from build123d import *

# Parameters (mm, degrees)
SKETCH1_R                      = 6.25
SKETCH1_R_2                    = 3.75
SKETCH1_R_3                    = 2.5
BOSS_EXTRUDE1_DEPTH            = 5
SKETCH2_R                      = 4
BOSS_EXTRUDE2_DEPTH            = 22.5
SKETCH3_R                      = 3
BOSS_EXTRUDE3_DEPTH            = 2
SKETCH4_R                      = 4
BOSS_EXTRUDE4_DEPTH            = 2
SKETCH6_W                      = 1.89865
SKETCH6_H                      = 5
F_6_CLEARANCE_HOLE1_AT_2_COUNT = 2
F_6_CLEARANCE_HOLE1_AT_2_PITCH = 7.75


with BuildPart() as part:
    # Sketch1 → Boss-Extrude1 (new body)
    # profile 1 of 15: a face of its own
    with BuildSketch(Plane(origin=(0, 0, 0), x_dir=(1, 0, 0), z_dir=(0, 1, 0))):
        Circle(SKETCH1_R)
    # profile 2 of 15: a face of its own
    with BuildSketch(Plane(origin=(0, 0, 0), x_dir=(1, 0, 0), z_dir=(0, 1, 0))):
        with Locations((-7.75, 0)):
            Circle(SKETCH1_R_2)
        with Locations((-7.75, 0)):
            Circle(SKETCH1_R_3, mode=Mode.SUBTRACT)
    # profile 3 of 15: a face of its own
    with BuildSketch(Plane(origin=(0, 0, 0), x_dir=(1, 0, 0), z_dir=(0, 1, 0))):
        Circle(SKETCH1_R)
    # profile 4 of 15: a face of its own
    with BuildSketch(Plane(origin=(0, 0, 0), x_dir=(1, 0, 0), z_dir=(0, 1, 0))):
        with Locations((-7.75, 0)):
            Circle(SKETCH1_R_2)
        with Locations((-7.75, 0)):
            Circle(SKETCH1_R_3, mode=Mode.SUBTRACT)
    # profile 5 of 15: a face of its own
    with BuildSketch(Plane(origin=(0, 0, 0), x_dir=(1, 0, 0), z_dir=(0, 1, 0))):
        with Locations((7.75, 0)):
            Circle(SKETCH1_R_2)
    # profile 6 of 15: a face of its own
    with BuildSketch(Plane(origin=(0, 0, 0), x_dir=(1, 0, 0), z_dir=(0, 1, 0))):
        Circle(SKETCH1_R)
    # profile 7 of 15: a face of its own
    with BuildSketch(Plane(origin=(0, 0, 0), x_dir=(1, 0, 0), z_dir=(0, 1, 0))):
        with Locations((-7.75, 0)):
            Circle(SKETCH1_R_2)
    # profile 8 of 15: a face of its own
    with BuildSketch(Plane(origin=(0, 0, 0), x_dir=(1, 0, 0), z_dir=(0, 1, 0))):
        with BuildLine():
            ThreePointArc((-5.487903226, -2.990889196), (-7.15425073, -3.702375293), (-8.959677419, -3.54953244))
            Line((-8.959677419, -3.54953244), (-2.016129032, -5.9158874))
            ThreePointArc((-2.016129032, -5.9158874), (-4.026975125, -4.77974595), (-5.487903226, -2.990889196))
        make_face()
    # profile 9 of 15: a face of its own
    with BuildSketch(Plane(origin=(0, 0, 0), x_dir=(1, 0, 0), z_dir=(0, 1, 0))):
        with BuildLine():
            ThreePointArc((5.487903226, -2.990889196), (4.026975125, -4.77974595), (2.016129032, -5.9158874))
            Line((2.016129032, -5.9158874), (8.959677419, -3.54953244))
            ThreePointArc((8.959677419, -3.54953244), (7.15425073, -3.702375293), (5.487903226, -2.990889196))
        make_face()
    # profile 10 of 15: a face of its own
    with BuildSketch(Plane(origin=(0, 0, 0), x_dir=(1, 0, 0), z_dir=(0, 1, 0))):
        Circle(SKETCH1_R)
    # profile 11 of 15: a face of its own
    with BuildSketch(Plane(origin=(0, 0, 0), x_dir=(1, 0, 0), z_dir=(0, 1, 0))):
        with Locations((7.75, 0)):
            Circle(SKETCH1_R_2)
        with Locations((7.75, 0)):
            Circle(SKETCH1_R_3, mode=Mode.SUBTRACT)
    # profile 12 of 15: a face of its own
    with BuildSketch(Plane(origin=(0, 0, 0), x_dir=(1, 0, 0), z_dir=(0, 1, 0))):
        with Locations((7.75, 0)):
            Circle(SKETCH1_R_2)
        with Locations((7.75, 0)):
            Circle(SKETCH1_R_3, mode=Mode.SUBTRACT)
    # profile 13 of 15: a face of its own
    with BuildSketch(Plane(origin=(0, 0, 0), x_dir=(1, 0, 0), z_dir=(0, 1, 0))):
        Circle(SKETCH1_R)
    # profile 14 of 15: a face of its own
    with BuildSketch(Plane(origin=(0, 0, 0), x_dir=(1, 0, 0), z_dir=(0, 1, 0))):
        with BuildLine():
            Line((8.959677419, 3.54953244), (2.016129032, 5.9158874))
            ThreePointArc((2.016129032, 5.9158874), (4.026975125, 4.77974595), (5.487903226, 2.990889196))
            ThreePointArc((5.487903226, 2.990889196), (7.15425073, 3.702375293), (8.959677419, 3.54953244))
        make_face()
    # profile 15 of 15: a face of its own
    with BuildSketch(Plane(origin=(0, 0, 0), x_dir=(1, 0, 0), z_dir=(0, 1, 0))):
        with BuildLine():
            Line((-2.016129032, 5.9158874), (-8.959677419, 3.54953244))
            ThreePointArc((-8.959677419, 3.54953244), (-7.15425073, 3.702375293), (-5.487903226, 2.990889196))
            ThreePointArc((-5.487903226, 2.990889196), (-4.026975125, 4.77974595), (-2.016129032, 5.9158874))
        make_face()
    extrude(amount=BOSS_EXTRUDE1_DEPTH)

    # Sketch2 → Boss-Extrude2 (add)
    with BuildSketch(Plane(origin=(0, 5, 0), x_dir=(1, 0, 0), z_dir=(0, 1, 0))):
        with Locations(Location((0, 0, 0), (0, 0, 90))):
            Circle(SKETCH2_R)
    extrude(amount=BOSS_EXTRUDE2_DEPTH)

    # Sketch3 → Boss-Extrude3 (add)
    with BuildSketch(Plane(origin=(0, 27.5, 0), x_dir=(1, 0, 0), z_dir=(0, 1, 0))):
        with Locations(Location((0, 0, 0), (0, 0, 270))):
            Circle(SKETCH3_R)
    extrude(amount=BOSS_EXTRUDE3_DEPTH)

    # Sketch4 → Boss-Extrude4 (add)
    with BuildSketch(Plane(origin=(0, 29.5, 0), x_dir=(1, 0, 0), z_dir=(0, 1, 0))):
        with Locations(Location((0, 0, 0), (0, 0, 90))):
            Circle(SKETCH4_R)
    extrude(amount=BOSS_EXTRUDE4_DEPTH)

    # Sketch6 → #6 Clearance Hole1 (revolve, cut)
    with BuildSketch(Plane(origin=(7.75, 5, 0), x_dir=(0, 0, 1), z_dir=(1, 0, 0))):
        with Locations((0.949325, 2.5)):
            Rectangle(SKETCH6_W, SKETCH6_H)
    f_6_clearance_hole1 = revolve(axis=Axis((7.75, 11.35, 0), (0, -1, 0)), mode=Mode.SUBTRACT)

    # #6 Clearance Hole1 at 2: #6 Clearance Hole1 ×2
    with Locations(*[(-i * F_6_CLEARANCE_HOLE1_AT_2_PITCH, 0, 0) for i in range(1, F_6_CLEARANCE_HOLE1_AT_2_COUNT)]):
        add(f_6_clearance_hole1, mode=Mode.SUBTRACT)


solid = part.part
Geometry check sheet. Reference: the model listing, model coordinates, mm. A direction names the side the tool comes from. Give positions to 0.01 mm unless a question says otherwise; leave off trailing zeros. Loops run counter-clockwise (first coordinate to the right, second up) from the corner with the lowest first, then second, coordinate; pieces in that order, holes last. Notation, with made-up numbers: M 22.5,27.5 L 45.5,27.5 A32 cw 45.5,65.5 Z; hole C 19,-33.75 d11. An arc over 180 degrees is marked long. Answer as a JSON object with one key per item and string values. Group by question number.
Item 1: Sectioned sample at B-B on x = 7.75. Record the boundary of the cut face in (y, z).
Item 2: Sectioned sample at A-A on z = 0. Record the boundary of the cut face in (x, y), plus the area to 3 significant figures.
Item 3: Sectioned sample at C-C on x = 0. Record the boundary of the cut face in (y, z).
Item 4: Sectioned sample at D-D on y = 19.5. Record the boundary of the cut face in (x, z), plus the area to 3 significant figures.
Item 5: Access from +Z, -Z, +X, -X, +Y, -Y to the whole of each face (thin tool, end or side, straight path). Record for faces 1 (the flat face through (-0.2, 5, -4.3)), 2 (the cylindrical face through (0.9, 28.49, 2.86)), 3 (the flat face through (0, 5, 0)).
Item 6: Material ranges on L1, parallel to X at y = 2.65, z = 0; L2, parallel to Y at x = 0.25, z = -3.5; L3, parallel to Y at x = -2.75, z = -3.75, recorded low to high.
Item 7: Gauge pin test, flat ends, axial feed: pin 1 (10 mm diameter, centred on x = 0.5, y = 25, fed in from +Z); pin 2 (1 mm diameter, centred on y = 15.5, z = -3.5, fed in from +X); pin 3 (5 mm diameter, centred on x = 6, y = 24, fed in from -Z). Record the tip position at first contact, or that the pin passes through.
Item 8: Mould release check, pull along Z, two halves, no side actions. Record for faces 4 (the flat face through (-5.537, 2.465, 4.716)), 5 (the cylindrical face through (-11.5, 2.5, -0.1)), 6 (the cylindrical face through (1.684, 2.465, 0.876)): pulls with the +Z half, pulls with the -Z half, needs draft (parallel to the pull), parting line crosses it, or undercut.
Findings below:
{
 "1": {"outline": "M 0,-3.96 L 5,-3.96 L 5,-1.9 L 0,-1.9 Z; M 0,1.9 L 5,1.9 L 5,3.96 L 0,3.96 Z"},
 "2": {"outline": "M -11.5,0 L -1.9,0 L -1.9,5 L 1.9,5 L 1.9,0 L 5.85,0 L 5.85,5 L 4,5 L 4,27.5 L 3,27.5 L 3,29.5 L 4,29.5 L 4,31.5 L -4,31.5 L -4,29.5 L -3,29.5 L -3,27.5 L -4,27.5 L -4,5 L -11.5,5 Z; M 9.65,0 L 11.5,0 L 11.5,5 L 9.65,5 Z", "area": "285 mm2"},
 "3": {"outline": "M 0,-6.25 L 5,-6.25 L 5,-4 L 27.5,-4 L 27.5,-3 L 29.5,-3 L 29.5,-4 L 31.5,-4 L 31.5,4 L 29.5,4 L 29.5,3 L 27.5,3 L 27.5,4 L 5,4 L 5,6.25 L 0,6.25 L 0,1.9 L 5,1.9 L 5,-1.9 L 0,-1.9 Z"},
 "4": {"outline": "C 0,0 d8", "area": "50.3 mm2"},
 "5": {"face 1": "+Y", "face 2": "none", "face 3": "-Y"},
 "6": {"L1": "-11.5 to -1.9, 1.9 to 5.85, 9.65 to 11.5", "L2": "0 to 27.5, 29.5 to 31.5", "L3": "0 to 5"},
 "7": {"pin 1": "z = 4", "pin 2": "x = 2.65", "pin 3": "z = -1.94"},
 "8": {"face 4": "pulls with the +Z half", "face 5": "parting line crosses it", "face 6": "undercut"}
}
